```python
from build123d import *

# Parameters (mm, degrees)
F1_DEPTH = 143.7894
F3_DEPTH = 143.7904
F5_DEPTH = 38.1


with BuildPart() as f1:
    # F0 (on Front) → F1 (new body)
    with BuildSketch(Plane.XZ):
        with BuildLine():
            Line((13.589, 10.3759), (-13.589, 10.3759))
            Line((-13.589, 10.3759), (-13.589, -12.2301))
            Line((-13.589, -12.2301), (-11.8745, -12.2301))
            Line((-11.8745, -12.2301), (-11.8745, -19.2151))
            ThreePointArc((-11.8745, -19.2151), (0, -28.7401), (11.8745, -19.2151))
            Line((11.8745, -19.2151), (11.8745, -12.2301))
            Line((11.8745, -12.2301), (13.589, -12.2301))
            Line((13.589, -12.2301), (13.589, 10.3759))
        make_face()
    extrude(amount=-F1_DEPTH)

    # F2 (on face) → F3 (cut, through all)
    with BuildSketch(Plane.XZ):
        with BuildLine():
            ThreePointArc((-10.541, 9.270239), (-5.299414, 10.098729), (0, 10.3759))
            ThreePointArc((0, 10.3759), (5.299414, 10.098729), (10.541, 9.270239))
            ThreePointArc((10.541, 9.270239), (12.298376, 6.870264), (13.589, 4.190239))
            Line((13.589, 4.190239), (13.589, 18.64491))
            Line((13.589, 18.64491), (-13.877228, 18.64491))
            Line((-13.877228, 18.64491), (-13.589, 4.190239))
            ThreePointArc((-13.589, 4.190239), (-12.298376, 6.870264), (-10.541, 9.270239))
        make_face()
    extrude(amount=-F3_DEPTH, mode=Mode.SUBTRACT)

    # F4 (on Top) → F5 (cut, symmetric)
    with BuildSketch(Plane.XY):
        with BuildLine():
            ThreePointArc((13.589, 1.851261), (0, 0), (-13.589, 1.851261))
            Line((-13.589, 1.851261), (-13.589, -7.918205))
            Line((-13.589, -7.918205), (13.589, -7.918205))
            Line((13.589, -7.918205), (13.589, 1.851261))
        make_face()
    extrude(amount=F5_DEPTH, both=True, mode=Mode.SUBTRACT)


solid = f1.part
```
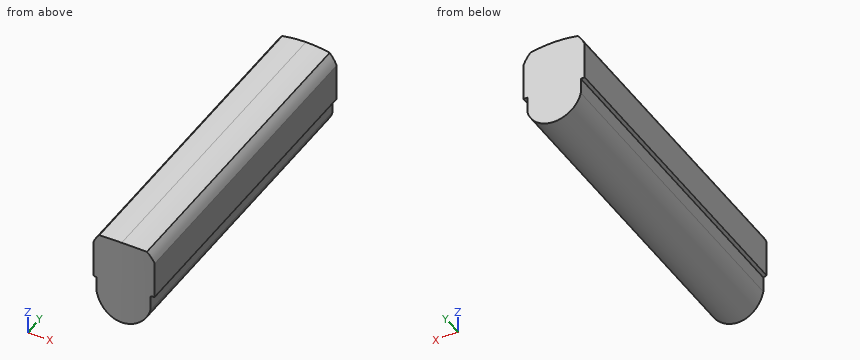
For this review, take the finished solid that the model builds, in its own axes (mm). Round coordinates to 2 decimals unless told otherwise and drop trailing zeros. Write each loop counter-clockwise with the first axis right and the second up, starting at its lowest first coordinate (ties: lowest second). Pieces come first, ordered by that corner, then holes.
1) Take a section at A-A on y = 82.5. Give the boundary of the cut face in (x, z).
Answer below:
outline: (-13.59, -12.23) - (-11.87, -12.23) - (-11.87, -19.22) arc R12.16 ccw to (11.87, -19.22) - (11.87, -12.23) - (13.59, -12.23) - (13.59, 4.19) arc R16.26 ccw to (10.54, 9.27) arc R50.8 ccw to (0, 10.38) arc R50.8 ccw to (-10.54, 9.27) arc R16.26 ccw to (-13.59, 4.19) - close
2) For line 1 along X through (y, z) = (37, -16); line 2 along Y through (x, z) = (11.75, -18.5); line 3 along Y through (x, z) = (-0.5, -8.5), list the stretches that pass through material, from the lowest coordinate up.
Answer below:
line 1: x = -11.87 to 11.87
line 2: y = 1.38 to 143.79
line 3: y = 0 to 143.79
3) Insertion check: pin 1 Ø12 at (y, z) = (101, -24.5) entering from -X; pin 2 Ø1.5 at (x, z) = (-10, -24) entering from -Y; pin 3 Ø2 at (x, y) = (9.5, 84.5) entering from -Z. Each pin has a flat end and moves straight along its axis. Give the tip position at first contact, or say it passes through.
Answer below:
pin 1: stops at x = -11.87
pin 2: stops at y = 0.85
pin 3: stops at z = -25.28
4) Take a section at C-C on z = 7.5. Give the boundary of the cut face in (x, y).
Answer below:
outline: (-11.9, 1.41) arc R50.8 ccw to (11.9, 1.41) - (11.9, 143.79) - (-11.9, 143.79) - close
5) Take a section at B-B on x = -6.75. Give the boundary of the cut face in (y, z), then the cut area to 3 significant figures.
Answer below:
outline: (0.45, -26.7) - (143.79, -26.7) - (143.79, 9.93) - (0.45, 9.93) - close
area: 5,250 mm2
